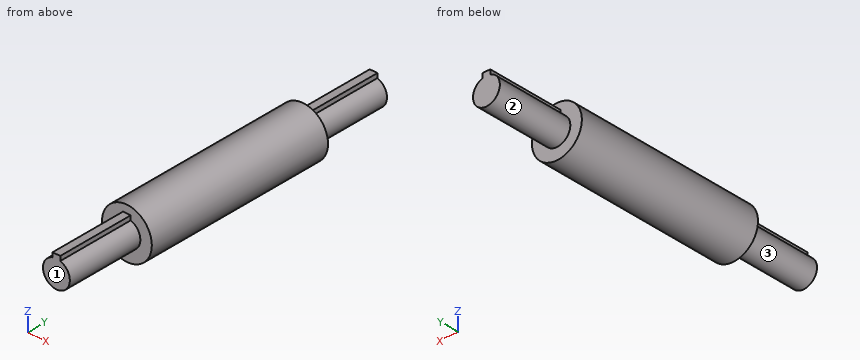
```python
from build123d import *

# Parameters (mm, degrees)
SKETCH1_R                = 3.25
BOSS_EXTRUDE1_DEPTH      = 25
SKETCH2_R                = 1.75
BOSS_EXTRUDE2_DEPTH      = 10
BOSS_EXTRUDE2_DEPTH_BACK = 35
BOSS_EXTRUDE3_START      = -45
SKETCH3_W                = 1
SKETCH3_H                = 1
BOSS_EXTRUDE3_DEPTH      = 45


with BuildPart() as part:
    # Sketch1 → Boss-Extrude1 (new body)
    with BuildSketch(Plane(origin=(0, 0, 0), x_dir=(1, 0, 0), z_dir=(0, 1, 0))):
        Circle(SKETCH1_R)
    extrude(amount=BOSS_EXTRUDE1_DEPTH)

    # Sketch2 → Boss-Extrude2 (add, two sides)
    with BuildSketch(Plane(origin=(0, 25, 0), x_dir=(1, 0, 0), z_dir=(0, 1, 0))) as boss_extrude2_sk:
        Circle(SKETCH2_R)
    extrude(amount=BOSS_EXTRUDE2_DEPTH)
    extrude(boss_extrude2_sk.sketch, amount=-BOSS_EXTRUDE2_DEPTH_BACK)

    # Sketch3 → Boss-Extrude3 (add)
    with BuildSketch(Plane.XZ.offset(10).offset(BOSS_EXTRUDE3_START)):
        with Locations((0, 1.75)):
            Rectangle(SKETCH3_W, SKETCH3_H)
    extrude(amount=BOSS_EXTRUDE3_DEPTH)


solid = part.part
```
Can you work these out from the model? Positions are in its coordinate system, mm. Face numbers are marked on the shaded views. A direction names the side the tool comes from. Coordinates: 2 decimals unless noted, no trailing zeros. Loops run counter-clockwise (first coordinate to the right, second up) from the corner with the lowest first, then second, coordinate; pieces in that order, holes last. Notation, with made-up numbers: (58.5, -22.5) -> (84.5, -22.5) arc R18 cw to (84.5, 10.5) -> close; hole circle Ø4 at (34, 37). An arc over 180 degrees is marked (long way). Answer as a JSON object with one key per item and string values.
1) Imagine slicing it at C-C (y = 21.5). Please give me the cut outline in (x, z), then the cut area to 3 significant figures.
Results:
{"outline": "circle Ø6.5 at (0, 0)", "area": "33.2 mm^2"}
2) For the marked faces 1, 2 and 3, which set-ups out of +Z, -Z, +X, -X, +Y, -Y let a thin tool reach every point of the face, with its end or its side?
Results:
{"face 1": "+Z, -Z, +X, -X, -Y", "face 2": "+Y", "face 3": "-Y"}
3) Imagine slicing it at A-A (z = 0). Please give me the cut outline in (x, y).
Results:
{"outline": "(-3.25, 0) -> (-1.75, 0) -> (-1.75, -10) -> (1.75, -10) -> (1.75, 0) -> (3.25, 0) -> (3.25, 25) -> (1.75, 25) -> (1.75, 35) -> (-1.75, 35) -> (-1.75, 25) -> (-3.25, 25) -> close"}
4) For P1, Ø1, axis at x = -2.5, z = -2.5, coming from the -Y side; P2, Ø0.5, axis at x = 0, y = 28.5, coming from the +Z side; P3, Ø0.5, axis at y = 31, z = 2, coming from the +X side, each with a flat end and sliding along its axis, tell me the tip position at first contact or that it passes through.
Results:
{"P1": "stops at y = 0", "P2": "stops at z = 2.25", "P3": "stops at x = 0.5"}
5) If I drill on line 1 (Z direction, x = 0, y = -1.5); line 2 (Y direction, x = -1.75, z = 2.5); line 3 (Z direction, x = 0.75, y = 33), over which ranges is the centre line in solid material (lowest first)?
Results:
{"line 1": "z = -1.75 to 2.25", "line 2": "y = 0 to 25", "line 3": "z = -1.58 to 1.58"}
6) Imagine slicing it at B-B (x = 0). Please give me the cut outline in (y, z), then the cut area to 4 significant figures.
Results:
{"outline": "(-10, -1.75) -> (0, -1.75) -> (0, -3.25) -> (25, -3.25) -> (25, -1.75) -> (35, -1.75) -> (35, 2.25) -> (25, 2.25) -> (25, 3.25) -> (0, 3.25) -> (0, 2.25) -> (-10, 2.25) -> close", "area": "242.5 mm^2"}
